Input: part model. Units: mm. Frame: model coordinates. A direction names the side the tool comes from. Coordinates: 2 decimals unless noted, no trailing zeros. Write each loop counter-clockwise with the first axis right and the second up, starting at its lowest first coordinate (ties: lowest second). Pieces come first, ordered by that corner, then holes. Notation, with made-up numbers: M 42,44.25 L 55,44.25 A30 ccw 55,73.25 Z; hole C 45.5,32.25 d6. An arc over 180 degrees is marked long. Use CSV: the item, a comma, the result in double quotes.
```python
from build123d import *

# Parameters (mm, degrees)
F0_R     = 11.2
F0_W     = 6.3229973894
F0_H     = 3.449
F1_DEPTH = 7
F2_R     = 1.5


# Not quite as in the source:
# - ends of sketch curves that miss each other by under 0.0002 mm in the source are joined


with BuildPart() as f1:
    # F0 (on Top) → F1 (new body)
    with BuildSketch(Plane.XY):
        Polygon((-3.3052028157, 17.9631426474), (3.0177945737, 17.9631426474), (8.6286484148, 17.9631426474), (17.2572757273, 32.9083635521), (8.628630128, 47.8536161306), (-8.628630128, 47.8536161306), (-17.2572757273, 32.9083635521), (-8.6286484148, 17.9631426474), align=None)
        with Locations((0, 32.9083055258)):
            Circle(F0_R, mode=Mode.SUBTRACT)
        Polygon((3.3052028157, -14.5141426474), (8.3797441645, -14.5141426474), (16.759488329, 0), (8.3797441645, 14.5141426474), (3.0177945737, 14.5141426474), (-3.3052028157, 14.5141426474), (-8.3797441645, 14.5141426474), (-16.759488329, 0), (-8.3797441645, -14.5141426474), (-3.0177945737, -14.5141426474), align=None)
        Circle(F0_R, mode=Mode.SUBTRACT)
        with Locations((-0.143704121, 16.2386426474)):
            Rectangle(F0_W, F0_H)
        Polygon((8.6286484148, -17.9630480707), (3.3052028157, -17.9630480707), (-3.0177945737, -17.9630480707), (-8.6286484148, -17.9630480707), (-17.2572757273, -32.9082689754), (-8.628630128, -47.8535215539), (8.628630128, -47.8535215539), (17.2572757273, -32.9082689754), align=None)
        with Locations((0, -32.9082109491)):
            Circle(F0_R, mode=Mode.SUBTRACT)
        with Locations((0.143704121, -16.2386426474)):
            Rectangle(F0_W, F0_H)
    extrude(amount=F1_DEPTH)

    # F2
    f2_edges = [f1.edges().sort_by_distance(p)[0] for p in [
        (-12.942953, 40.38099, 7),
        (0, 47.853616, 7),
        (12.942953, 40.38099, 7),
        (12.942962, 25.435753, 7),
        (-12.942962, 25.435753, 7),
        (-12.569616, 7.257071, 7),
        (12.569616, -7.257071, 7),
        (-12.569616, -7.257071, 7),
        (-12.942962, -25.435659, 7),
        (12.942962, -25.435659, 7),
        (12.942953, -40.380895, 7),
        (0, -47.853522, 7),
        (-12.942953, -40.380895, 7),
        (12.569616, 7.257071, 7),
        (-12.942953, -40.380895, 0),
        (0, -47.853522, 0),
        (12.942953, -40.380895, 0),
        (12.942962, -25.435659, 0),
        (-12.942962, -25.435659, 0),
        (-12.569616, -7.257071, 0),
        (12.569616, -7.257071, 0),
        (12.569616, 7.257071, 0),
        (-12.569616, 7.257071, 0),
        (-12.942962, 25.435753, 0),
        (-12.942953, 40.38099, 0),
        (12.942953, 40.38099, 0),
        (0, 47.853616, 0),
        (12.942962, 25.435753, 0),
    ]]
    fillet(f2_edges, radius=F2_R)


solid = f1.part
```
1. Section A-A (x = 0). Return loops of the section in (y, z).
Resolved:
outline,"M -47.85,1.5 A1.5 ccw -46.35,0 L -44.11,0 L -44.11,7 L -46.35,7 A1.5 ccw -47.85,5.5 Z; M -21.71,0 L -11.2,0 L -11.2,7 L -21.71,7 Z; M 11.2,0 L 21.71,0 L 21.71,7 L 11.2,7 Z; M 44.11,0 L 46.35,0 A1.5 ccw 47.85,1.5 L 47.85,5.5 A1.5 ccw 46.35,7 L 44.11,7 Z"
2. Access query for faces 1 (the cylindrical face through (-12.29, 25.16, 0.45)), 2 (the cylindrical face through (-12.419, -25.384, 6.549)), 3 (the cylindrical face through (12.044, -7.311, 6.549)), 4 (the flat face through (-3.305, 16, 3)), 5 (the flat face through (13, 40.28, 3.47)). Directions: +Z, -Z, +X, -X, +Y, -Y. A direction counts if a zero-diameter tool reaches every point of the face in a straight line with its end or side. Return the directions, or none.
Resolved:
face 1,"-Z, -X"
face 2,"+Z, -X"
face 3,"+Z, +X"
face 4,"+Z, -Z, -X"
face 5,"+Z, -Z, +X, +Y"
3. Material intervals for line 1 (Y direction, x = 0, z = 2); line 2 (Y direction, x = 0, z = 6.5); line 3 (Y direction, x = -13, z = 4.25), sorted ascending. Write a range as [from, to].
Resolved:
line 1,"y = [-47.85, -44.11], [-21.71, -11.2], [11.2, 21.71], [44.11, 47.85]"
line 2,"y = [-47.47, -44.11], [-21.71, -11.2], [11.2, 21.71], [44.11, 47.47]"
line 3,"y = [-40.28, -25.53], [-6.51, 6.51], [25.53, 40.28]"
4. Section B-B (z = 3.75). State how many separate pieces and enclosed holes the cut face has, then the cut area to 3 significant figures.
Resolved:
separate pieces,"1"
enclosed holes,"3"
area,"1,140 mm^2"
5. Mould query, pull axis Y, two halves, no side actions, for faces 6 (the flat face through (-12.88, 40.49, 3.47)), 7 (the cylindrical face through (-8.255, 40.478, 3.451)), 8 (the cylindrical face through (-12.51, -40.27, 0.45)). Classes: pulls with the +Y half, pulls with the -Y half, needs draft (parallel to the pull), parting line crosses it, or undercut.
Resolved:
face 6,"pulls with the +Y half"
face 7,"undercut"
face 8,"pulls with the -Y half"
6. Contact query for flat-ended pins moving along their axis: pin 1 Ø1 at (y, z) = (16, 3.5) entering from -X; pin 2 Ø1.7 at (y, z) = (-15.5, 4.5) entering from +X; pin 3 Ø4 at (y, z) = (-9, 1.5) entering from +X; pin 4 Ø20 at (x, y) = (0, 0) entering from -Z. Output: stop coordinate, or through.
Resolved:
pin 1,"stops at x = -3.31"
pin 2,"stops at x = 3.31"
pin 3,"stops at x = 12.72"
pin 4,"passes through"
